The model under review builds one solid part; all positions refer to its coordinate system, in mm. A direction names the side the tool comes from. Coordinates: 2 decimals unless noted, no trailing zeros. Loops run counter-clockwise (first coordinate to the right, second up) from the corner with the lowest first, then second, coordinate; pieces in that order, holes last. Notation, with made-up numbers: M 61.5,-20 L 67.5,-20 A20 ccw 67.5,2 Z; hole C -38.5,34.5 d3. An arc over 180 degrees is marked long. Write item = value, one per line. Start each with the question number.
Q1. We need section B-B on z = -32.5. Give the boundary of the cut face in (x, y) (3 decimals).
Q2. Wall thickness on probe 1 along X at (y, z) = (-2, -62); probe 2 along X at (y, z) = (-2.25, -62.5); probe 3 along Z at (x, y) = (-63, -10.5): over which ranges is each line inside the solid? List them lowest first.
Q3. Clearance check with flat-ended pins moving along their axes: pin 1 Ø6.5 at (y, z) = (-4.5, -9) entering from +X; pin 2 Ø4 at (y, z) = (-4, -12.5) entering from +X; pin 3 Ø1.5 at (x, z) = (-66, -0.5) entering from -Y. State where each tip first meets the part, or that it passes through.
Q4. Mouldability with a two-part tool opening along X and no side actions: class faces 3 (the face through (-17.895, -6.261, -80.587)), 4 (the face through (67, -6.35, 0)), 5 (the face through (-20, 0, 1)) as released by +X, released by -X, zero draft, split by the parting line, or undercut.
Q5. We need section D-D on x = -21. Give the boundary of the cut face in (y, z), and give its area (3 significant figures).
Q6. For faces 1 (the face through (-43.335, -6, 0)), 2 (the face through (64.51, -9.48, 0.11)), list the 3-axis set-ups (+Z, -Z, +X, -X, +Y, -Y) from which the entire face can be reached by the end or side of a thin tool; tool diameter is ignored.
Q7. We need section A-A on z = -14.5. Count the separate pieces of the cut face and the enclosed holes in it, and give its area (3 significant figures).
from build123d import *

# Parameters (mm, degrees)
F0_R     = 82.55
F1_DEPTH = 6.35
F2_R     = 82.55
F2_R_2   = 2.54
F3_DEPTH = 6.35


with BuildPart() as f1:
    # F0 (on Front) → F1 (new body)
    with BuildSketch(Plane.XZ):
        Circle(F0_R)
        with BuildLine():
            Line((3.175, 53.897562), (3.175, -60.402438))
            ThreePointArc((3.175, -60.402438), (2.245064, -62.647502), (0, -63.577438))
            ThreePointArc((0, -63.577438), (-2.245064, -62.647502), (-3.175, -60.402438))
            Line((-3.175, -60.402438), (-3.175, 53.897562))
            ThreePointArc((-3.175, 53.897562), (-2.245064, 56.142626), (0, 57.072562))
            ThreePointArc((0, 57.072562), (2.245064, 56.142626), (3.175, 53.897562))
        make_face(mode=Mode.SUBTRACT)
        with BuildLine():
            Line((-49.684873, -19.05), (-49.684873, 19.05))
            ThreePointArc((-49.684873, 19.05), (-48.754937, 21.295064), (-46.509873, 22.225))
            ThreePointArc((-46.509873, 22.225), (-44.264809, 21.295064), (-43.334873, 19.05))
            Line((-43.334873, 19.05), (-43.334873, -19.05))
            ThreePointArc((-43.334873, -19.05), (-44.264809, -21.295064), (-46.509873, -22.225))
            ThreePointArc((-46.509873, -22.225), (-48.754937, -21.295064), (-49.684873, -19.05))
        make_face(mode=Mode.SUBTRACT)
        with BuildLine():
            Line((-33.980241, -25.7175), (-33.980241, 25.7175))
            ThreePointArc((-33.980241, 25.7175), (-33.050305, 27.962564), (-30.805241, 28.8925))
            ThreePointArc((-30.805241, 28.8925), (-28.560177, 27.962564), (-27.630241, 25.7175))
            Line((-27.630241, 25.7175), (-27.630241, -25.7175))
            ThreePointArc((-27.630241, -25.7175), (-28.560177, -27.962564), (-30.805241, -28.8925))
            ThreePointArc((-30.805241, -28.8925), (-33.050305, -27.962564), (-33.980241, -25.7175))
        make_face(mode=Mode.SUBTRACT)
        with BuildLine():
            Line((-17.973594, -44.45), (-17.973594, 44.45))
            ThreePointArc((-17.973594, 44.45), (-17.043658, 46.695064), (-14.798594, 47.625))
            ThreePointArc((-14.798594, 47.625), (-12.55353, 46.695064), (-11.623594, 44.45))
            Line((-11.623594, 44.45), (-11.623594, -44.45))
            ThreePointArc((-11.623594, -44.45), (-12.55353, -46.695064), (-14.798594, -47.625))
            ThreePointArc((-14.798594, -47.625), (-17.043658, -46.695064), (-17.973594, -44.45))
        make_face(mode=Mode.SUBTRACT)
        with BuildLine():
            ThreePointArc((11.623594, 44.45), (12.55353, 46.695064), (14.798594, 47.625))
            ThreePointArc((14.798594, 47.625), (17.043658, 46.695064), (17.973594, 44.45))
            Line((17.973594, 44.45), (17.973594, -44.45))
            ThreePointArc((17.973594, -44.45), (17.043658, -46.695064), (14.798594, -47.625))
            ThreePointArc((14.798594, -47.625), (12.55353, -46.695064), (11.623594, -44.45))
            Line((11.623594, -44.45), (11.623594, 44.45))
        make_face(mode=Mode.SUBTRACT)
        with BuildLine():
            ThreePointArc((33.980241, -25.7175), (33.050305, -27.962564), (30.805241, -28.8925))
            ThreePointArc((30.805241, -28.8925), (28.560177, -27.962564), (27.630241, -25.7175))
            Line((27.630241, -25.7175), (27.630241, 25.7175))
            ThreePointArc((27.630241, 25.7175), (28.560177, 27.962564), (30.805241, 28.8925))
            ThreePointArc((30.805241, 28.8925), (33.050305, 27.962564), (33.980241, 25.7175))
            Line((33.980241, 25.7175), (33.980241, -25.7175))
        make_face(mode=Mode.SUBTRACT)
        with BuildLine():
            ThreePointArc((43.334873, 19.05), (44.264809, 21.295064), (46.509873, 22.225))
            ThreePointArc((46.509873, 22.225), (48.754937, 21.295064), (49.684873, 19.05))
            Line((49.684873, 19.05), (49.684873, -19.05))
            ThreePointArc((49.684873, -19.05), (48.754937, -21.295064), (46.509873, -22.225))
            ThreePointArc((46.509873, -22.225), (44.264809, -21.295064), (43.334873, -19.05))
            Line((43.334873, -19.05), (43.334873, 19.05))
        make_face(mode=Mode.SUBTRACT)
    extrude(amount=F1_DEPTH)

    # F2 (on face) → F3 (join)
    with BuildSketch(Plane.XZ.offset(6.35)):
        Circle(F2_R)
        with BuildLine():
            Line((-3.175, -60.402438), (-3.175, 53.897562))
            ThreePointArc((-3.175, 53.897562), (0, 57.072562), (3.175, 53.897562))
            Line((3.175, 53.897562), (3.175, -60.402438))
            ThreePointArc((3.175, -60.402438), (0, -63.577438), (-3.175, -60.402438))
        make_face(mode=Mode.SUBTRACT)
        with Locations((-67.046702, 0)):
            Circle(F2_R_2, mode=Mode.SUBTRACT)
        with BuildLine():
            Line((-43.334873, 19.05), (-43.334873, -19.05))
            ThreePointArc((-43.334873, -19.05), (-46.509873, -22.225), (-49.684873, -19.05))
            Line((-49.684873, -19.05), (-49.684873, 19.05))
            ThreePointArc((-49.684873, 19.05), (-46.509873, 22.225), (-43.334873, 19.05))
        make_face(mode=Mode.SUBTRACT)
        with BuildLine():
            Line((-27.630241, 25.7175), (-27.630241, -25.7175))
            ThreePointArc((-27.630241, -25.7175), (-30.805241, -28.8925), (-33.980241, -25.7175))
            Line((-33.980241, -25.7175), (-33.980241, 25.7175))
            ThreePointArc((-33.980241, 25.7175), (-30.805241, 28.8925), (-27.630241, 25.7175))
        make_face(mode=Mode.SUBTRACT)
        with BuildLine():
            Line((-11.623594, 44.45), (-11.623594, -44.45))
            ThreePointArc((-11.623594, -44.45), (-14.798594, -47.625), (-17.973594, -44.45))
            Line((-17.973594, -44.45), (-17.973594, 44.45))
            ThreePointArc((-17.973594, 44.45), (-14.798594, 47.625), (-11.623594, 44.45))
        make_face(mode=Mode.SUBTRACT)
        with BuildLine():
            ThreePointArc((17.973594, -44.45), (14.798594, -47.625), (11.623594, -44.45))
            Line((11.623594, -44.45), (11.623594, 44.45))
            ThreePointArc((11.623594, 44.45), (14.798594, 47.625), (17.973594, 44.45))
            Line((17.973594, 44.45), (17.973594, -44.45))
        make_face(mode=Mode.SUBTRACT)
        with BuildLine():
            ThreePointArc((27.630241, 25.7175), (30.805241, 28.8925), (33.980241, 25.7175))
            Line((33.980241, 25.7175), (33.980241, -25.7175))
            ThreePointArc((33.980241, -25.7175), (30.805241, -28.8925), (27.630241, -25.7175))
            Line((27.630241, -25.7175), (27.630241, 25.7175))
        make_face(mode=Mode.SUBTRACT)
        with BuildLine():
            ThreePointArc((49.684873, -19.05), (46.509873, -22.225), (43.334873, -19.05))
            Line((43.334873, -19.05), (43.334873, 19.05))
            ThreePointArc((43.334873, 19.05), (46.509873, 22.225), (49.684873, 19.05))
            Line((49.684873, 19.05), (49.684873, -19.05))
        make_face(mode=Mode.SUBTRACT)
        with Locations((67.046702, 0)):
            Circle(F2_R_2, mode=Mode.SUBTRACT)
    extrude(amount=F3_DEPTH)


solid = f1.part
Returned:
q1.outline = M -75.883,-12.7 L -17.974,-12.7 L -17.974,0 L -75.883,0 Z; M -11.624,-12.7 L -3.175,-12.7 L -3.175,0 L -11.624,0 Z; M 3.175,-12.7 L 11.624,-12.7 L 11.624,0 L 3.175,0 Z; M 17.974,-12.7 L 75.883,-12.7 L 75.883,0 L 17.974,0 Z
q2.probe_1 = -54.5 to -2.74, 2.74 to 54.5
q2.probe_2 = -53.93 to -2.38, 2.38 to 53.93
q2.probe_3 = -53.34 to 53.34
q3.pin_1 = 82.35
q3.pin_2 = 81.88
q3.pin_3 = -6.35
q4.face_3 = split by the parting line
q4.face_4 = undercut
q4.face_5 = zero draft
q5.outline = M -12.7,-79.83 L 0,-79.83 L 0,79.83 L -12.7,79.83 Z
q5.area = 2,030 mm^2
q6.face_1 = +Y, -Y
q6.face_2 = -Y
q7.separate_pieces = 8
q7.enclosed_holes = 0
q7.area = 1,500 mm^2
